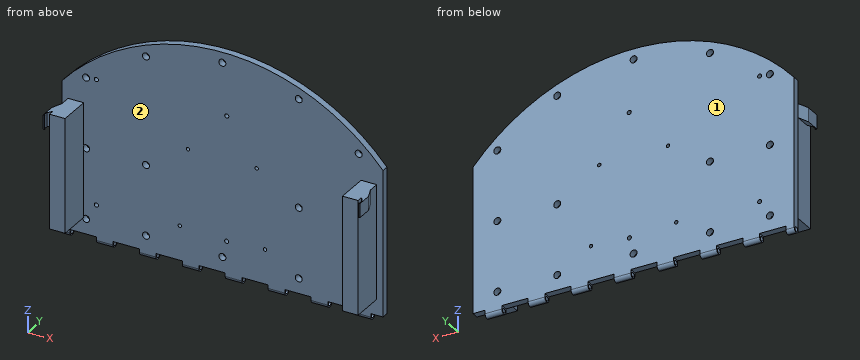
```python
from build123d import *

# Parameters (mm, degrees)
BOSS_EXTRUDE1_DEPTH      = 5.08
SKETCH2_W                = 11.329576632
SKETCH2_H                = 83
BOSS_EXTRUDE2_DEPTH      = 23.622
BOSS_EXTRUDE3_DEPTH      = 154.884757
BOSS_EXTRUDE3_DEPTH_BACK = 154.884757
SKETCH4_W                = 19.05
SKETCH4_H                = 5.08
CUT_EXTRUDE2_DEPTH       = 5.08
SKETCH5_R                = 1.25
CUT_EXTRUDE3_DEPTH       = 5.08
SKETCH6_W                = 87.378176536
SKETCH6_H                = 116.226136144
CUT_EXTRUDE5_DEPTH       = 5.08
SKETCH7_R                = 2.54
CUT_EXTRUDE6_DEPTH       = 5.08
SKETCH8_R                = 1.55
CUT_EXTRUDE7_DEPTH       = 224.79
BOSS_EXTRUDE4_DEPTH      = 10.16
BOSS_EXTRUDE5_DEPTH      = 10.16
SKETCH12_R               = 1.5
CUT_EXTRUDE8_DEPTH       = 5.08


with BuildPart() as part:
    # Sketch1 → Boss-Extrude1 (new body)
    with BuildSketch(Plane(origin=(0, 0, 0), x_dir=(1, 0, 0), z_dir=(0, 1, 0))):
        with BuildLine():
            ThreePointArc((154.94, 0), (154.926188711, 2.068731835), (154.884757307, 4.137094858))
            Line((154.884757307, 4.137094858), (-154.884757307, 4.137094858))
            ThreePointArc((-154.884757307, 4.137094858), (-2.068731835, -154.926188711), (154.94, 0))
        make_face()
    extrude(amount=BOSS_EXTRUDE1_DEPTH)

    # Sketch2 → Boss-Extrude2 (add)
    with BuildSketch(Plane(origin=(0, 0, 0), x_dir=(-1, 0, 0), z_dir=(0, -1, 0))):
        with Locations((-106.53347234, -48.850905142)):
            Rectangle(SKETCH2_W, SKETCH2_H)
        with Locations((106.53347234, -48.850905142)):
            Rectangle(SKETCH2_W, SKETCH2_H)
    extrude(amount=BOSS_EXTRUDE2_DEPTH)

    # Sketch3 → Boss-Extrude3 (add, two sides)
    with BuildSketch(Plane(origin=(0, 0, 0), x_dir=(0, 0, -1), z_dir=(1, 0, 0))) as boss_extrude3_sk:
        with BuildLine():
            ThreePointArc((9.217094858, 2.54), (8.473146082, 4.336051224), (6.677094858, 5.08))
            Line((6.677094858, 5.08), (6.677094858, 0))
            ThreePointArc((6.677094858, 0), (8.473146082, 0.743948776), (9.217094858, 2.54))
        make_face()
        with BuildLine():
            Line((6.677094858, 0), (6.677094858, 5.08))
            ThreePointArc((6.677094858, 5.08), (4.881043633, 4.336051224), (4.137094858, 2.54))
            ThreePointArc((4.137094858, 2.54), (4.881043633, 0.743948776), (6.677094858, 0))
        make_face()
        with BuildLine():
            Line((6.677094858, 5.08), (4.137094858, 5.08))
            Line((4.137094858, 5.08), (4.137094858, 2.54))
            ThreePointArc((4.137094858, 2.54), (4.881043633, 4.336051224), (6.677094858, 5.08))
        make_face()
        with BuildLine():
            ThreePointArc((6.677094858, 0), (4.881043633, 0.743948776), (4.137094858, 2.54))
            Line((4.137094858, 2.54), (4.137094858, 0))
            Line((4.137094858, 0), (6.677094858, 0))
        make_face()
    extrude(amount=BOSS_EXTRUDE3_DEPTH)
    extrude(boss_extrude3_sk.sketch, amount=-BOSS_EXTRUDE3_DEPTH_BACK)

    # Sketch4 → Cut-Extrude2 (cut)
    with BuildSketch(Plane(origin=(0, 5.08, 0), x_dir=(1, 0, 0), z_dir=(0, 1, 0))):
        with Locations((-132.429084549, 6.677094858)):
            Rectangle(SKETCH4_W, SKETCH4_H)
        with Locations((-101.187084549, 6.677094858)):
            Rectangle(SKETCH4_W, SKETCH4_H)
        with Locations((-69.945084549, 6.677094858)):
            Rectangle(SKETCH4_W, SKETCH4_H)
        with Locations((-38.703084549, 6.677094858)):
            Rectangle(SKETCH4_W, SKETCH4_H)
        with Locations((-7.461084549, 6.677094858)):
            Rectangle(SKETCH4_W, SKETCH4_H)
        with Locations((23.780915451, 6.677094858)):
            Rectangle(SKETCH4_W, SKETCH4_H)
        with Locations((55.022915451, 6.677094858)):
            Rectangle(SKETCH4_W, SKETCH4_H)
        with Locations((86.264915451, 6.677094858)):
            Rectangle(SKETCH4_W, SKETCH4_H)
        with Locations((117.506915451, 6.677094858)):
            Rectangle(SKETCH4_W, SKETCH4_H)
        with Locations((148.748915451, 6.677094858)):
            Rectangle(SKETCH4_W, SKETCH4_H)
    extrude(amount=-CUT_EXTRUDE2_DEPTH, mode=Mode.SUBTRACT)

    # Sketch5 → Cut-Extrude3 (cut)
    with BuildSketch(Plane(origin=(0, 5.08, 0), x_dir=(1, 0, 0), z_dir=(0, 1, 0))):
        with Locations((-31, -20.830897674)):
            Circle(SKETCH5_R)
        with Locations((-25, -77.830897674)):
            Circle(SKETCH5_R)
        with Locations((31, -20.830897674)):
            Circle(SKETCH5_R)
        with Locations((25, -77.830897674)):
            Circle(SKETCH5_R)
    extrude(amount=-CUT_EXTRUDE3_DEPTH, mode=Mode.SUBTRACT)

    # Sketch6 → Cut-Extrude5 (cut)
    with BuildSketch(Plane(origin=(0, 5.08, 0), x_dir=(1, 0, 0), z_dir=(0, 1, 0))):
        with Locations((160.497172817, -43.682192054)):
            Rectangle(SKETCH6_W, SKETCH6_H)
        with Locations((-160.497172817, -43.682192054)):
            Rectangle(SKETCH6_W, SKETCH6_H)
    extrude(amount=-CUT_EXTRUDE5_DEPTH, mode=Mode.SUBTRACT)

    # Sketch7 → Cut-Extrude6 (cut)
    with BuildSketch(Plane(origin=(0, 5.08, 0), x_dir=(1, 0, 0), z_dir=(0, 1, 0))):
        with Locations((0, -147.32)):
            Circle(SKETCH7_R)
        with Locations((0, -6.788708839)):
            Circle(SKETCH7_R)
        with Locations((55.543786685, -136.448049311)):
            Circle(SKETCH7_R)
        with Locations((-55.543786685, -136.448049311)):
            Circle(SKETCH7_R)
        with Locations((-99.114141025, -108.993437642)):
            Circle(SKETCH7_R)
        with Locations((-99.114141025, -6.788708839)):
            Circle(SKETCH7_R)
        with Locations((99.114141025, -6.788708839)):
            Circle(SKETCH7_R)
        with Locations((-55.543786685, -6.788708839)):
            Circle(SKETCH7_R)
        with Locations((55.543786685, -6.788708839)):
            Circle(SKETCH7_R)
        with Locations((99.114141025, -108.993437642)):
            Circle(SKETCH7_R)
        with Locations((-99.114141025, -57.89107324)):
            Circle(SKETCH7_R)
        with Locations((99.114141025, -57.89107324)):
            Circle(SKETCH7_R)
        with Locations((55.543786685, -57.89107324)):
            Circle(SKETCH7_R)
        with Locations((-55.543786685, -57.89107324)):
            Circle(SKETCH7_R)
    extrude(amount=-CUT_EXTRUDE6_DEPTH, mode=Mode.SUBTRACT)

    # Sketch8 → Cut-Extrude7 (cut)
    with BuildSketch(Plane(origin=(107.981915451, 0, 0), x_dir=(0, 0, -1), z_dir=(1, 0, 0))):
        with Locations((6.677094858, 2.54)):
            Circle(SKETCH8_R)
    extrude(amount=-CUT_EXTRUDE7_DEPTH, mode=Mode.SUBTRACT)

    # Sketch9 → Boss-Extrude4 (add)
    with BuildSketch(Plane.XY.offset(90.350905142)):
        Polygon((115.246260656, -15.633482352), (112.198260656, -15.633482352), (112.198260656, -19.189482352), (114.611260656, -22.745482352), (114.611260656, -25.77835243), (114.103260656, -25.886331163), (114.103260656, -26.46263354), (114.611260656, -26.570612273), (115.246260656, -26.570612273), align=None)
        Polygon((-114.611260656, -25.77835243), (-114.611260656, -22.745482352), (-112.198260656, -19.189482352), (-112.198260656, -15.633482352), (-115.246260656, -15.633482352), (-115.246260656, -26.570612273), (-114.611260656, -26.570612273), (-114.103260656, -26.46263354), (-114.103260656, -25.886331163), align=None)
    extrude(amount=-BOSS_EXTRUDE4_DEPTH)

    # Sketch11 → Boss-Extrude5 (add)
    with BuildSketch(Plane.XY.offset(90.350905142)):
        Polygon((112.198260656, -7.816741176), (115.246260656, -15.633482352), (112.198260656, -15.633482352), align=None)
        Polygon((-115.246260656, -15.633482352), (-112.198260656, -15.633482352), (-112.198260656, -7.816741176), align=None)
    extrude(amount=-BOSS_EXTRUDE5_DEPTH)

    # Sketch12 → Cut-Extrude8 (cut)
    with BuildSketch(Plane(origin=(0, 5.08, 0), x_dir=(1, 0, 0), z_dir=(0, 1, 0))):
        with Locations((-91.646084549, -18.920905142)):
            Circle(SKETCH12_R)
        with Locations((-91.646084549, -109.710905142)):
            Circle(SKETCH12_R)
        with Locations((3.207915451, -109.710905142)):
            Circle(SKETCH12_R)
        with Locations((3.094524951, -19.034295642)):
            Circle(SKETCH12_R)
    extrude(amount=-CUT_EXTRUDE8_DEPTH, mode=Mode.SUBTRACT)


solid = part.part
```
Check sheet for the modelled part. Datum: model origin and axes. Units: mm. Face numbers are marked on the shaded views. Give positions to 0.01 mm unless a question says otherwise; leave off trailing zeros. Order: outer loops, then holes, each group sorted by start corner. A loop starts at its lowest first (then second) coordinate and runs counter-clockwise, first axis right, second up. Notation, with made-up numbers: M -4.75,25 L 52.25,25 A22 cw 52.25,42 Z; hole C 19,15.25 d2. An arc over 180 degrees is marked long. Answer in a Markdown table with one row per item.
1) Release check for a two-part mould opening along X. For the marked faces 1 and 2 record: +X half, -X half, draft (parallel to the pull), parting line (faces both ways), or undercut.
Filled sheet:
| item | result |
|---|---|
| face 1 | draft |
| face 2 | undercut |
2) Thickness scan on L1, parallel to X at y = -17.5, z = 23; L2, parallel to Y at x = -76, z = 13.5; L3, parallel to Z at x = 104, y = -9. Record the ranges inside material, lowest first. Write a range as [from, to].
Filled sheet:
| item | result |
|---|---|
| L1 | x = [-112.2, -100.87], [100.87, 112.2] |
| L2 | y = [0, 5.08] |
| L3 | z = [7.35, 90.35] |
3) Cross-section at B-B, the plane z = 147.32. Enter the section's corners in (x, y).
Filled sheet:
| item | result |
|---|---|
| outline | M -47.99,0 L -2.54,0 L -2.54,5.08 L -47.99,5.08 Z; M 2.54,0 L 47.99,0 L 47.99,5.08 L 2.54,5.08 Z |
4) Cross-section at A-A, the plane y = -5.5. Enter the section's corners in (x, z).
Filled sheet:
| item | result |
|---|---|
| outline | M -112.2,7.35 L -100.87,7.35 L -100.87,90.35 L -112.2,90.35 Z; M 100.87,7.35 L 112.2,7.35 L 112.2,90.35 L 100.87,90.35 Z |
5) Gauge pin test, flat ends, axial feed: P1, Ø5.5, axis at x = 104, y = -9, coming from the -Z side; P2, Ø4, axis at y = -21.5, z = 73.5, coming from the -X side; P3, Ø2.5, axis at x = -114.5, y = -18, coming from the -Z side. Record the tip position at first contact, or that the pin passes through.
Filled sheet:
| item | result |
|---|---|
| P1 | stops at z = 7.35 |
| P2 | stops at x = -112.2 |
| P3 | stops at z = 80.19 |
6) Cross-section at C-C, the plane z = 71.5. Enter the section's corners in (x, y), plus the area to 3 significant figures.
Filled sheet:
| item | result |
|---|---|
| outline | M -116.81,0 L -112.2,0 L -112.2,-23.62 L -100.87,-23.62 L -100.87,0 L 100.87,0 L 100.87,-23.62 L 112.2,-23.62 L 112.2,0 L 116.81,0 L 116.81,5.08 L -116.81,5.08 Z |
| area | 1,720 mm2 |
7) Cross-section at D-D, the plane x = 84. Enter the section's corners in (y, z).
Filled sheet:
| item | result |
|---|---|
| outline | M 0,-4.14 L 5.08,-4.14 L 5.08,130.19 L 0,130.19 Z |
